Solid Edge part; units mm, degrees
sketch "Sketch1" plane through (0, 0, 0) normal (0, -1, 0) x (1, 0, 0)
  line L0 (0, -6) -> (1, -6)
  line L1 (1, -6) -> (1, -0.501)
  line L2 (1, -0.501) -> (0.87, -0.101)
  line L3 (0.87, -0.101) -> (0.87, 0)
  line L4 (0.87, 0) -> (2, 0)
  line L5 (2, 0) -> (1.8863, 1.3)
  line L6 (1.8863, 1.3) -> (0, 1.3)
  dimension "D1" = 0.87
  dimension "D2" = 1
  dimension "D3" = 1.8863
revolve "RevolvedProtrusion1" add sketch "Sketch1" angle 360 about axis through (0, 0, 6) along (0, 0, -1)
fillet "Round_1" radius 0.6 1 edges at (-1.8863, 0, 1.3)
sketch "Sketch2" plane through (0, 0, 0) normal (0, -1, 0) x (1, 0, 0)
  line L0 (-0.25, 1.3) -> (-0.25, 0.8)
  line L1 (-0.25, 0.8) -> (0.25, 0.8)
  line L2 (0.25, 0.8) -> (0.25, 1.3)
  line L3 (0.25, 1.3) -> (-0.25, 1.3)
  dimension "D1" = 0.25
  dimension "D2" = 0.25
extrude "ExtrudedCutout_1" cut sketch "Sketch2" along normal mid plane 4
cosmetic_thread "Thread_1" thread depth 5.499
fillet "Round_2" radius 0.1 1 edges at (-0.87, 0, 0)
chamfer "Chamfer_1" distance 0.0012 angle 30 1 edges at (-1, 0, -6) measured on face at (0.6867, 0.6467, -6)
properties material "Steel"
CAD build for the part. Positions are in the model's coordinates, mm. A direction names the side the tool comes from. Coordinates: 2 decimals unless noted, no trailing zeros. Loops run counter-clockwise (first coordinate to the right, second up) from the corner with the lowest first, then second, coordinate; pieces in that order, holes last. Notation, with made-up numbers: (1.25, 68.5) - (22.25, 68.5) arc R31 ccw to (22.25, 102.5) - close; hole circle Ø5 at (-21, 50). An arc over 180 degrees is marked (long way). Write item = value, one per line. Start each with the question number.
Q1. Drill centre lines: L1, parallel to X at y = -1.45, z = 0.5; L2, parallel to Z at x = 0.4, y = 1.3; L3, parallel to Z at x = 0, y = -0.6. Where is each one in solid material? Low to high.
Q2. Which spindle directions (+Z, -Z, +X, -X, +Y, -Y) get a long thin tool onto all of the face, cutting with end or side? Do faces 1 (the conical face through (-0.423, 1.907, 0.538)), 2 (the cylindrical face through (0, -1, -3)). Say none if no direction does.
Q3. Cut at C-C, the plane z = -2.25. List the corners of the cut face in (x, y), then the cut area to 3 significant figures.
Q4. Cut at D-D, the plane z = 0.25. List the corners of the cut face in (x, y).
Q5. Flat gauge pins, fed straight in: pin 1 Ø1.5 at (y, z) = (-1, -4) entering from +X; pin 2 Ø1.2 at (x, y) = (-0.5, 1) entering from -Z; pin 3 Ø1.5 at (x, z) = (-1, 0.5) entering from +Y. Where does each tip first touch, or does it go through?
Computed:
q1.L1 = -1.31 to 1.31
q1.L2 = 0 to 1.3
q1.L3 = -6 to 0.8
q2.face_1 = +Z
q2.face_2 = -Z
q3.outline = circle Ø2 at (0, 0)
q3.area = 3.14 mm²
q4.outline = circle Ø3.96 at (0, 0)
q5.pin_1 = 0.97
q5.pin_2 = -6
q5.pin_3 = 1.96
